from build123d import *

# Parameters (mm, degrees)
BOSS_EXTRUDE1_DEPTH                           = 8.5
FILLET1_R                                     = 1
SKETCH2_W                                     = 83
SKETCH2_H                                     = 214
CUT_EXTRUDE1_DEPTH                            = 7
SKETCH3_W                                     = 97
SKETCH3_H                                     = 214
CUT_EXTRUDE2_DEPTH                            = 7
FILLET2_R                                     = 2
CSK_FOR_0_FLAT_HEAD_MACHINE_SCREW1_AT_2_COUNT = 2
CSK_FOR_0_FLAT_HEAD_MACHINE_SCREW1_AT_2_PITCH = 22.666666667
CSK_FOR_0_FLAT_HEAD_MACHINE_SCREW1_AT_3_COUNT = 2
CSK_FOR_0_FLAT_HEAD_MACHINE_SCREW1_AT_3_PITCH = 45.333333333
CSK_FOR_0_FLAT_HEAD_MACHINE_SCREW1_AT_4_COUNT = 2
CSK_FOR_0_FLAT_HEAD_MACHINE_SCREW1_AT_4_PITCH = 68
CSK_FOR_0_FLAT_HEAD_MACHINE_SCREW1_AT_5_COUNT = 2
CSK_FOR_0_FLAT_HEAD_MACHINE_SCREW1_AT_5_PITCH = 90.666666667
CSK_FOR_0_FLAT_HEAD_MACHINE_SCREW1_AT_6_COUNT = 2
CSK_FOR_0_FLAT_HEAD_MACHINE_SCREW1_AT_6_PITCH = 113.333333333
CSK_FOR_0_FLAT_HEAD_MACHINE_SCREW1_AT_7_COUNT = 2
CSK_FOR_0_FLAT_HEAD_MACHINE_SCREW1_AT_7_PITCH = 136
CSK_FOR_0_FLAT_HEAD_MACHINE_SCREW1_AT_8_COUNT = 2
CSK_FOR_0_FLAT_HEAD_MACHINE_SCREW1_AT_8_PITCH = 158.666666667
CSK_FOR_0_FLAT_HEAD_MACHINE_SCREW1_AT_9_COUNT = 2
CSK_FOR_0_FLAT_HEAD_MACHINE_SCREW1_AT_9_PITCH = 181.333333333
CSK_FOR_0_FLAT_HEAD_MACHINE_SCREW1_AT_1_COUNT = 2
CSK_FOR_0_FLAT_HEAD_MACHINE_SCREW1_AT_1_PITCH = 204


with BuildPart() as part:
    # Sketch1 → Boss-Extrude1 (new body)
    with BuildSketch(Plane.XY):
        Polygon((-41.5, -107), (41.5, -107), (41.5, -113.5), (50, -113.5), (50, -107), (50, 107), (50, 113.5), (41.5, 113.5), (41.5, 107), (-41.5, 107), (-41.5, 113.5), (-50, 113.5), (-50, 107), (-50, -107), (-50, -113.5), (-41.5, -113.5), align=None)
    extrude(amount=BOSS_EXTRUDE1_DEPTH)

    # Fillet1
    fillet1_edges = [part.edges().sort_by_distance(p)[0] for p in [
        (50, 0, 0),
        (45.75, -113.5, 0),
        (-45.75, -113.5, 0),
        (-50, 0, 0),
        (-45.75, 113.5, 0),
        (-45.75, 113.5, 8.5),
        (45.75, 113.5, 0),
        (50, -113.5, 4.25),
        (41.5, -113.5, 4.25),
        (-41.5, -113.5, 4.25),
        (-50, -113.5, 4.25),
        (-50, 113.5, 4.25),
        (-41.5, 113.5, 4.25),
        (41.5, 113.5, 4.25),
        (50, 113.5, 4.25),
        (-45.75, -113.5, 8.5),
        (45.75, -113.5, 8.5),
        (45.75, 113.5, 8.5),
    ]]
    fillet(fillet1_edges, radius=FILLET1_R)

    # Sketch2 → Cut-Extrude1 (cut)
    with BuildSketch(Plane.XY.offset(8.5)):
        Rectangle(SKETCH2_W, SKETCH2_H)
    extrude(amount=-CUT_EXTRUDE1_DEPTH, mode=Mode.SUBTRACT)

    # Sketch3 → Cut-Extrude2 (cut)
    with BuildSketch(Plane.XY.offset(8.5)):
        Rectangle(SKETCH3_W, SKETCH3_H)
    extrude(amount=-CUT_EXTRUDE2_DEPTH, mode=Mode.SUBTRACT)

    # Fillet2
    fillet2_edges = [part.edges().sort_by_distance(p)[0] for p in [
        (-48.5, 107, 5),
        (48.5, -107, 5),
        (-48.5, -107, 5),
        (48.5, 107, 5),
    ]]
    fillet(fillet2_edges, radius=FILLET2_R)

    # Sketch4 → CSK for #0 Flat Head Machine Screw1 (revolve, cut)
    with BuildSketch(Plane(origin=(-50, 102, 4.25), x_dir=(0, 0, 1), z_dir=(0, 1, 0))):
        Polygon((0, 0), (0, 3.83616509), (0.889, 3.302), (0.889, 0.969878135), (1.7321022, 0), align=None)
    csk_for_0_flat_head_machine_screw1 = revolve(axis=Axis((-56.35, 102, 4.25), (1, 0, 0)), mode=Mode.SUBTRACT)

    # CSK for #0 Flat Head Machine Screw1 at 2: CSK for #0 Flat Head Machine Screw1 ×2
    with Locations(*[(0, -i * CSK_FOR_0_FLAT_HEAD_MACHINE_SCREW1_AT_2_PITCH, 0) for i in range(1, CSK_FOR_0_FLAT_HEAD_MACHINE_SCREW1_AT_2_COUNT)]):
        add(csk_for_0_flat_head_machine_screw1, mode=Mode.SUBTRACT)

    # CSK for #0 Flat Head Machine Screw1 at 3: CSK for #0 Flat Head Machine Screw1 ×2
    with Locations(*[(0, -i * CSK_FOR_0_FLAT_HEAD_MACHINE_SCREW1_AT_3_PITCH, 0) for i in range(1, CSK_FOR_0_FLAT_HEAD_MACHINE_SCREW1_AT_3_COUNT)]):
        add(csk_for_0_flat_head_machine_screw1, mode=Mode.SUBTRACT)

    # CSK for #0 Flat Head Machine Screw1 at 4: CSK for #0 Flat Head Machine Screw1 ×2
    with Locations(*[(0, -i * CSK_FOR_0_FLAT_HEAD_MACHINE_SCREW1_AT_4_PITCH, 0) for i in range(1, CSK_FOR_0_FLAT_HEAD_MACHINE_SCREW1_AT_4_COUNT)]):
        add(csk_for_0_flat_head_machine_screw1, mode=Mode.SUBTRACT)

    # CSK for #0 Flat Head Machine Screw1 at 5: CSK for #0 Flat Head Machine Screw1 ×2
    with Locations(*[(0, -i * CSK_FOR_0_FLAT_HEAD_MACHINE_SCREW1_AT_5_PITCH, 0) for i in range(1, CSK_FOR_0_FLAT_HEAD_MACHINE_SCREW1_AT_5_COUNT)]):
        add(csk_for_0_flat_head_machine_screw1, mode=Mode.SUBTRACT)

    # CSK for #0 Flat Head Machine Screw1 at 6: CSK for #0 Flat Head Machine Screw1 ×2
    with Locations(*[(0, -i * CSK_FOR_0_FLAT_HEAD_MACHINE_SCREW1_AT_6_PITCH, 0) for i in range(1, CSK_FOR_0_FLAT_HEAD_MACHINE_SCREW1_AT_6_COUNT)]):
        add(csk_for_0_flat_head_machine_screw1, mode=Mode.SUBTRACT)

    # CSK for #0 Flat Head Machine Screw1 at 7: CSK for #0 Flat Head Machine Screw1 ×2
    with Locations(*[(0, -i * CSK_FOR_0_FLAT_HEAD_MACHINE_SCREW1_AT_7_PITCH, 0) for i in range(1, CSK_FOR_0_FLAT_HEAD_MACHINE_SCREW1_AT_7_COUNT)]):
        add(csk_for_0_flat_head_machine_screw1, mode=Mode.SUBTRACT)

    # CSK for #0 Flat Head Machine Screw1 at 8: CSK for #0 Flat Head Machine Screw1 ×2
    with Locations(*[(0, -i * CSK_FOR_0_FLAT_HEAD_MACHINE_SCREW1_AT_8_PITCH, 0) for i in range(1, CSK_FOR_0_FLAT_HEAD_MACHINE_SCREW1_AT_8_COUNT)]):
        add(csk_for_0_flat_head_machine_screw1, mode=Mode.SUBTRACT)

    # CSK for #0 Flat Head Machine Screw1 at 9: CSK for #0 Flat Head Machine Screw1 ×2
    with Locations(*[(0, -i * CSK_FOR_0_FLAT_HEAD_MACHINE_SCREW1_AT_9_PITCH, 0) for i in range(1, CSK_FOR_0_FLAT_HEAD_MACHINE_SCREW1_AT_9_COUNT)]):
        add(csk_for_0_flat_head_machine_screw1, mode=Mode.SUBTRACT)

    # CSK for #0 Flat Head Machine Screw1 at 1: CSK for #0 Flat Head Machine Screw1 ×2
    with Locations(*[(0, -i * CSK_FOR_0_FLAT_HEAD_MACHINE_SCREW1_AT_1_PITCH, 0) for i in range(1, CSK_FOR_0_FLAT_HEAD_MACHINE_SCREW1_AT_1_COUNT)]):
        add(csk_for_0_flat_head_machine_screw1, mode=Mode.SUBTRACT)

    # Mirror1: CSK for #0 Flat Head Machine Screw1 across plane
    add(csk_for_0_flat_head_machine_screw1.mirror(Plane(origin=(0, 0, 0), x_dir=(0, 0, 1), z_dir=(1, 0, 0))), mode=Mode.SUBTRACT)

    # Mirror1 copy 1 sketch → Mirror1 copy 1 (revolve, cut)
    with BuildSketch(Plane(origin=(50, 79.333333333, 4.25), x_dir=(0, 0, 1), z_dir=(0, 1, 0))):
        Polygon((0, 0), (0, -3.83616509), (0.889, -3.302), (0.889, -0.969878135), (1.7321022, 0), align=None)
    revolve(axis=Axis((56.35, 79.333333333, 4.25), (1, 0, 0)), mode=Mode.SUBTRACT)

    # Mirror1 copy 2 sketch → Mirror1 copy 2 (revolve, cut)
    with BuildSketch(Plane(origin=(50, 56.666666667, 4.25), x_dir=(0, 0, 1), z_dir=(0, 1, 0))):
        Polygon((0, 0), (0, -3.83616509), (0.889, -3.302), (0.889, -0.969878135), (1.7321022, 0), align=None)
    revolve(axis=Axis((56.35, 56.666666667, 4.25), (1, 0, 0)), mode=Mode.SUBTRACT)

    # Mirror1 copy 3 sketch → Mirror1 copy 3 (revolve, cut)
    with BuildSketch(Plane(origin=(50, 34, 4.25), x_dir=(0, 0, 1), z_dir=(0, 1, 0))):
        Polygon((0, 0), (0, -3.83616509), (0.889, -3.302), (0.889, -0.969878135), (1.7321022, 0), align=None)
    revolve(axis=Axis((56.35, 34, 4.25), (1, 0, 0)), mode=Mode.SUBTRACT)

    # Mirror1 copy 4 sketch → Mirror1 copy 4 (revolve, cut)
    with BuildSketch(Plane(origin=(50, 11.333333333, 4.25), x_dir=(0, 0, 1), z_dir=(0, 1, 0))):
        Polygon((0, 0), (0, -3.83616509), (0.889, -3.302), (0.889, -0.969878135), (1.7321022, 0), align=None)
    revolve(axis=Axis((56.35, 11.333333333, 4.25), (1, 0, 0)), mode=Mode.SUBTRACT)

    # Mirror1 copy 5 sketch → Mirror1 copy 5 (revolve, cut)
    with BuildSketch(Plane(origin=(50, -11.333333333, 4.25), x_dir=(0, 0, 1), z_dir=(0, 1, 0))):
        Polygon((0, 0), (0, -3.83616509), (0.889, -3.302), (0.889, -0.969878135), (1.7321022, 0), align=None)
    revolve(axis=Axis((56.35, -11.333333333, 4.25), (1, 0, 0)), mode=Mode.SUBTRACT)

    # Mirror1 copy 6 sketch → Mirror1 copy 6 (revolve, cut)
    with BuildSketch(Plane(origin=(50, -34, 4.25), x_dir=(0, 0, 1), z_dir=(0, 1, 0))):
        Polygon((0, 0), (0, -3.83616509), (0.889, -3.302), (0.889, -0.969878135), (1.7321022, 0), align=None)
    revolve(axis=Axis((56.35, -34, 4.25), (1, 0, 0)), mode=Mode.SUBTRACT)

    # Mirror1 copy 7 sketch → Mirror1 copy 7 (revolve, cut)
    with BuildSketch(Plane(origin=(50, -56.666666667, 4.25), x_dir=(0, 0, 1), z_dir=(0, 1, 0))):
        Polygon((0, 0), (0, -3.83616509), (0.889, -3.302), (0.889, -0.969878135), (1.7321022, 0), align=None)
    revolve(axis=Axis((56.35, -56.666666667, 4.25), (1, 0, 0)), mode=Mode.SUBTRACT)

    # Mirror1 copy 8 sketch → Mirror1 copy 8 (revolve, cut)
    with BuildSketch(Plane(origin=(50, -79.333333333, 4.25), x_dir=(0, 0, 1), z_dir=(0, 1, 0))):
        Polygon((0, 0), (0, -3.83616509), (0.889, -3.302), (0.889, -0.969878135), (1.7321022, 0), align=None)
    revolve(axis=Axis((56.35, -79.333333333, 4.25), (1, 0, 0)), mode=Mode.SUBTRACT)

    # Mirror1 copy 9 sketch → Mirror1 copy 9 (revolve, cut)
    with BuildSketch(Plane(origin=(50, -102, 4.25), x_dir=(0, 0, 1), z_dir=(0, 1, 0))):
        Polygon((0, 0), (0, -3.83616509), (0.889, -3.302), (0.889, -0.969878135), (1.7321022, 0), align=None)
    revolve(axis=Axis((56.35, -102, 4.25), (1, 0, 0)), mode=Mode.SUBTRACT)


solid = part.part
Input: part model. Units: mm. Frame: model coordinates. A direction names the side the tool comes from. Give positions to 0.01 mm unless a question says otherwise; leave off trailing zeros. Write each loop counter-clockwise with the first axis right and the second up, starting at its lowest first coordinate (ties: lowest second). Pieces come first, ordered by that corner, then holes. Notation, with made-up numbers: M 80.25,87.5 L 105.25,87.5 A19 cw 105.25,122.5 Z; hole C -16,0 d3. An arc over 180 degrees is marked long. Write item = value, one per line. Start each with the question number.
1) Material intervals for line 1 along X through (y, z) = (-35, 7.25); line 2 along Z through (x, y) = (-48.6, -102); line 3 along Z through (x, y) = (-18, 103), sorted ascending. Write a range as [from, to].
2) Reachability of faces 5 (the flat face through (46, -113.5, 4)), 6 (the flat face through (-44, 107, 5)), 7 (the flat face through (41.5, -110, 4)), 8 (the flat face through (-41.5, 110, 4)) from +Z, -Z, +X, -X, +Y, -Y: full face, straight path, thin tool, end or side. Return the list, or none.
3) Cut plane A-A on y = 64. Return the cut outline in (x, z).
4) First-contact query: pin 1 Ø3 at (y, z) = (34, 4.25) entering from -X; pin 2 Ø0.8 at (x, z) = (13.5, 1) entering from +Y; pin 3 Ø1.6 at (y, z) = (11.33, 4.25) entering from +X; pin 4 Ø5 at (x, z) = (-38, 3.5) entering from -Y. Flat tips, straight axial feed; report the tip coordinate or a pass-through.
5) Cut plane B-B on x = -29. Return the cut outline in (y, z), then the cut area to 3 significant figures.
6) Draft query along Y for faces 1 (the flat face through (-46, 113.5, 4)), 2 (the flat face through (-48.5, -1, 5)), 3 (the flat face through (44, 107, 5)), 4 (the flat face through (-41.5, -110, 4)). Return one class per face: +Y half, -Y half, draft (parallel to the pull), parting line (faces both ways), or undercut.
Solved:
q1.line_1 = [-50, -48.5], [48.5, 50]
q1.line_2 = [0, 3.36], [5.14, 8.5]
q1.line_3 = [0, 1.5]
q2.face_5 = +Z, -Z, +X, -X, -Y
q2.face_6 = +Z
q2.face_7 = +Z, -Z, -Y
q2.face_8 = +Z, -Z, +Y
q3.outline = M -50,1 A1 ccw -49,0 L 49,0 A1 ccw 50,1 L 50,8.5 L 48.5,8.5 L 48.5,1.5 L -48.5,1.5 L -48.5,8.5 L -50,8.5 Z
q4.pin_1 = -49.73
q4.pin_2 = 107
q4.pin_3 = through
q4.pin_4 = -107
q5.outline = M -107,0 L 107,0 L 107,1.5 L -107,1.5 Z
q5.area = 321 mm2
q6.face_1 = +Y half
q6.face_2 = undercut
q6.face_3 = undercut
q6.face_4 = draft
